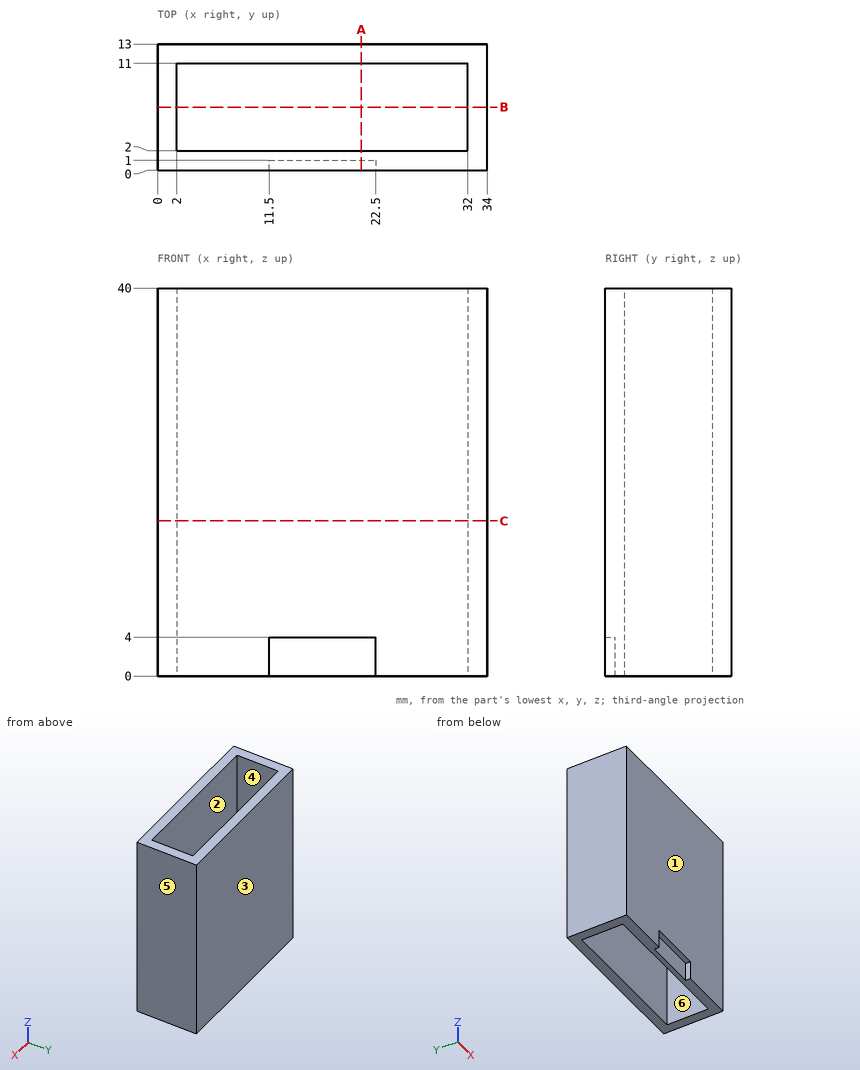
Answer from the drawing. Dimensions are ordinates in mm from the lowest x, y and z of the part. A direction names the side the tool comes from. Coordinates: 2 decimals unless noted, no trailing zeros. Write each loop counter-clockwise with the first axis right and the second up, starting at its lowest first coordinate (ties: lowest second). Pieces come first, ordered by that corner, then holes. Notation, with made-up numbers: (86, 59.25) - (121, 59.25) arc R8 cw to (121, 68.25) - close; hole circle Ø8 at (7.5, 36). An arc over 180 degrees is marked (long way). Return JSON: item names as keys, results as strings. Group by question number.
Q1. Find the intervals of material crossed by line 1 along X through (y, z) = (10.75, 12); line 2 along Y through (x, z) = (5.5, 20.5); line 3 along Y through (x, z) = (20.5, 3), in increasing order. Write a range as [from, to].
Q2. Which of the six approach directions +Z, -Z, +X, -X, +Y, -Y give full straight-line access (tool end or side, diameter ignored) to the marked faces 1 and 2?
Q3. Flat-ended cylindrical pins translate along their axes: pin 1 Ø4.5 at (y, z) = (6, 10.5) entering from -X; pin 2 Ø2 at (x, z) = (18.5, 2.5) entering from -Y; pin 3 Ø0.8 at (x, y) = (15, 0.5) entering from -Z. Find the tip coordinate at first contact, or state that the pin passes through.
Q4. The part is cut by section A-A on x = 21. Write down the section's boundary in (y, z), and give its area (3 significant figures).
Q5. The part is cut by section B-B on y = 6.5. Write down the section's boundary in (x, z).
Q6. For a pull along X with two mould halves and no side action, classify the marked faces 3, 4, 5 and 6 as +X half, -X half, draft (parallel to the pull), parting line (faces both ways), or undercut.
Q7. The part is cut by section C-C on z = 16. Write down the section's boundary in (x, y).
Evaluation:
{
 "1": {"line 1": "x = [0, 2], [32, 34]", "line 2": "y = [0, 2], [11, 13]", "line 3": "y = [1, 2], [11, 13]"},
 "2": {"face 1": "+Z, -Z, +X, -X, -Y", "face 2": "+Z, -Z"},
 "3": {"pin 1": "stops at x = 0", "pin 2": "stops at y = 1", "pin 3": "stops at z = 4"},
 "4": {"outline": "(0, 4) - (1, 4) - (1, 0) - (2, 0) - (2, 40) - (0, 40) - close; (11, 0) - (13, 0) - (13, 40) - (11, 40) - close", "area": "156 mm2"},
 "5": {"outline": "(0, 0) - (2, 0) - (2, 40) - (0, 40) - close; (32, 0) - (34, 0) - (34, 40) - (32, 40) - close"},
 "6": {"face 3": "draft", "face 4": "undercut", "face 5": "+X half", "face 6": "undercut"},
 "7": {"outline": "(0, 0) - (34, 0) - (34, 13) - (0, 13) - close; hole (2, 2) - (32, 2) - (32, 11) - (2, 11) - close"}
}
